Build history of the part. All positions in model axes, mm. A direction names the side the tool comes from. Give positions to 0.01 mm unless a question says otherwise; leave off trailing zeros. Loops run counter-clockwise (first coordinate to the right, second up) from the corner with the lowest first, then second, coordinate; pieces in that order, holes last. Notation, with made-up numbers: M 56.5,51 L 103.5,51 A34 cw 103.5,89 Z; hole C 35.5,-29.5 d3. An arc over 180 degrees is marked long. Put each result on its own line as item: value.
```python
from build123d import *

# Parameters (mm, degrees)
SKETCH24_W           = 25.1
SKETCH24_H           = 29.6
BOSS_EXTRUDE8_DEPTH  = 7
SKETCH26_W           = 9
SKETCH26_H           = 7
BOSS_EXTRUDE9_DEPTH  = 5
SKETCH27_W           = 9
SKETCH27_H           = 5
BOSS_EXTRUDE10_DEPTH = 174
SKETCH28_W           = 25.1
SKETCH28_H           = 34.6
BOSS_EXTRUDE11_DEPTH = 7
SKETCH29_W           = 16.1
SKETCH29_H           = 5
CUT_EXTRUDE8_DEPTH   = 15
SKETCH32_R           = 1.1
CUT_EXTRUDE11_DEPTH  = 29
SKETCH33_R           = 1.1
CUT_EXTRUDE13_DEPTH  = 21
SKETCH35_W           = 12
SKETCH35_H           = 5
BOSS_EXTRUDE12_DEPTH = 126
SKETCH38_R           = 3.1
CUT_EXTRUDE14_DEPTH  = 126


with BuildPart() as part:
    # Sketch24 → Boss-Extrude8 (new body)
    with BuildSketch(Plane.XY):
        with Locations((12.55, 14.8)):
            Rectangle(SKETCH24_W, SKETCH24_H)
    extrude(amount=BOSS_EXTRUDE8_DEPTH)

    # Sketch26 → Boss-Extrude9 (add)
    with BuildSketch(Plane(origin=(0, 29.6, 0), x_dir=(1, 0, 0), z_dir=(0, 1, 0))):
        with Locations((20.6, -3.5)):
            Rectangle(SKETCH26_W, SKETCH26_H)
    extrude(amount=BOSS_EXTRUDE9_DEPTH)

    # Sketch27 → Boss-Extrude10 (add)
    with BuildSketch(Plane(origin=(0, 0, 0), x_dir=(-1, 0, 0), z_dir=(0, 0, -1))):
        with Locations((-20.6, 32.1)):
            Rectangle(SKETCH27_W, SKETCH27_H)
    extrude(amount=BOSS_EXTRUDE10_DEPTH)

    # Sketch28 → Boss-Extrude11 (add)
    with BuildSketch(Plane(origin=(0, 0, -174), x_dir=(-1, 0, 0), z_dir=(0, 0, -1))):
        with Locations((-12.55, 17.3)):
            Rectangle(SKETCH28_W, SKETCH28_H)
    extrude(amount=BOSS_EXTRUDE11_DEPTH)

    # Sketch29 → Cut-Extrude8 (cut)
    with BuildSketch(Plane.XY.offset(-174)):
        with Locations((8.05, 32.1)):
            Rectangle(SKETCH29_W, SKETCH29_H)
    extrude(amount=-CUT_EXTRUDE8_DEPTH, mode=Mode.SUBTRACT)

    # Sketch32 → Cut-Extrude11 (cut)
    with BuildSketch(Plane(origin=(0, 0, -181), x_dir=(-1, 0, 0), z_dir=(0, 0, -1))):
        with Locations((-20.1, 5)):
            Circle(SKETCH32_R)
        with BuildLine():
            ThreePointArc((-6.6, 5), (-10.554058454, 14.545941546), (-20.1, 18.5))
            ThreePointArc((-20.1, 18.5), (-21.65, 20.05), (-20.1, 21.6))
            ThreePointArc((-20.1, 21.6), (-8.362027432, 16.737972568), (-3.5, 5))
            ThreePointArc((-3.5, 5), (-5.05, 3.45), (-6.6, 5))
        make_face()
    extrude(amount=-CUT_EXTRUDE11_DEPTH, mode=Mode.SUBTRACT)

    # Sketch33 → Cut-Extrude13 (cut)
    with BuildSketch(Plane.XY.offset(7)):
        with Locations((20.1, 5)):
            Circle(SKETCH33_R)
        with BuildLine():
            ThreePointArc((6.6, 5), (10.554058454, 14.545941546), (20.1, 18.5))
            ThreePointArc((20.1, 18.5), (21.65, 20.05), (20.1, 21.6))
            ThreePointArc((20.1, 21.6), (8.362027432, 16.737972568), (3.5, 5))
            ThreePointArc((3.5, 5), (5.05, 3.45), (6.6, 5))
        make_face()
    extrude(amount=-CUT_EXTRUDE13_DEPTH, mode=Mode.SUBTRACT)

    # Sketch35 → Boss-Extrude12 (add)
    with BuildSketch(Plane(origin=(25.1, 0, 0), x_dir=(0, 0, -1), z_dir=(1, 0, 0))):
        with Locations((-1, 32.1)):
            Rectangle(SKETCH35_W, SKETCH35_H)
    extrude(amount=BOSS_EXTRUDE12_DEPTH)

    # Sketch38 → Cut-Extrude14 (cut)
    with BuildSketch(Plane(origin=(0, 34.6, 0), x_dir=(1, 0, 0), z_dir=(0, 1, 0))):
        with Locations((142.6, -1)):
            Circle(SKETCH38_R)
        with Locations((94.6, -1)):
            Circle(SKETCH38_R)
    extrude(amount=-CUT_EXTRUDE14_DEPTH, mode=Mode.SUBTRACT)


solid = part.part
```
Q1. Mould opens along X. For faces 6 (the flat face through (12, 15, 0)), 7 (the flat face through (16.1, 32, -86)), 8 (the cylindrical face through (10.45, 14.44, 3.55)) say: pulls with the +X half, pulls with the -X half, needs draft (parallel to the pull), parting line crosses it, or undercut.
Here are the results:
face 6: needs draft
face 7: pulls with the -X half
face 8: undercut
Q2. Tool access for faces 1 (the flat face through (13, 15, -174)), 2 (the cylindrical face through (10.45, 14.44, -177.55)), 3 (the flat face through (23, 34.6, -45)), 4 (the flat face through (8, 29.6, 3)), 5 (the flat face through (25.1, 31, -106)): list every direction of +Z, -Z, +X, -X, +Y, -Y with a clear straight run to the whole face (end or side of a thin tool).
Here are the results:
face 1: +X, -X, -Y
face 2: +Z, -Z
face 3: +Z, -Z, +X, -X, +Y
face 4: +Z, -Z, -X, +Y
face 5: -Z, +X, +Y, -Y
Q3. Probe line 1 (X direction, y = 31, z = 1); line 2 (Y direction, x = 20, z = 2); line 3 (Z direction, x = 17.5, y = 7.5). List the from-to ranges inside material, lowest first. Write a range as from..to.
Here are the results:
line 1: 16.1..91.5, 97.7..139.5, 145.7..151.1
line 2: 0..3.9, 6.1..18.5, 21.6..34.6
line 3: -181..-174, 0..7
Q4. Slice it at D-D (x = 67). List the corners of the cut face in (y, z), and give its area (3 significant figures).
Here are the results:
outline: M 29.6,-5 L 34.6,-5 L 34.6,7 L 29.6,7 Z
area: 60.0 mm²
Q5. Slice it at B-B (y = 15). List the corners of the cut face in (x, z).
Here are the results:
outline: M 0,-181 L 6.85,-181 L 6.85,-174 L 0,-174 Z; M 0,0 L 6.85,0 L 6.85,7 L 0,7 Z; M 11.03,-181 L 25.1,-181 L 25.1,-174 L 11.03,-174 Z; M 11.03,0 L 25.1,0 L 25.1,7 L 11.03,7 Z
Q6. Slice it at A-A (x = 142.6). List the corners of the cut face in (y, z).
Here are the results:
outline: M 29.6,-5 L 34.6,-5 L 34.6,-2.1 L 29.6,-2.1 Z; M 29.6,4.1 L 34.6,4.1 L 34.6,7 L 29.6,7 Z
Q7. Slice it at C-C (z = -17.5). List the corners of the cut face in (x, y), and give its area (3 significant figures).
Here are the results:
outline: M 16.1,29.6 L 25.1,29.6 L 25.1,34.6 L 16.1,34.6 Z
area: 45.0 mm²
Q8. Drop flat-ended pins along their axis: pin 1 Ø3.5 at (x, z) = (9, -176.5) entering from +Y; pin 2 Ø4 at (x, y) = (119, 32.5) entering from -Z; pin 3 Ø4 at (y, z) = (31, -43) entering from -X. Give the stop position or say it passes through.
Here are the results:
pin 1: y = 29.6
pin 2: z = -5
pin 3: x = 16.1
